Verification items for the finished model (mm, model axes). A direction names the side the tool comes from. Give positions to 0.01 mm unless a question says otherwise; leave off trailing zeros. Loops run counter-clockwise (first coordinate to the right, second up) from the corner with the lowest first, then second, coordinate; pieces in that order, holes last. Notation, with made-up numbers: M 82,-22.5 L 97,-22.5 A36 cw 97,15.5 Z; hole C 1,43.5 d8. An arc over 180 degrees is marked long. Use a Markdown table: item, result.
from build123d import *

# Parameters (mm, degrees)
SKETCH1_R           = 125
BOSS_EXTRUDE1_DEPTH = 6
SKETCH2_R           = 2.5
CUT_EXTRUDE1_DEPTH  = 6
SKETCH3_R           = 12.5
CUT_EXTRUDE2_DEPTH  = 6
SKETCH5_R           = 2.5
CUT_EXTRUDE4_DEPTH  = 10
SKETCH7_R           = 1
CUT_EXTRUDE7_DEPTH  = 10
SKETCH8_R           = 2
CUT_EXTRUDE8_DEPTH  = 10
SKETCH9_R           = 1.25
CUT_EXTRUDE9_DEPTH  = 10
SKETCH10_R          = 8
CUT_EXTRUDE10_DEPTH = 10


with BuildPart() as part:
    # Sketch1 → Boss-Extrude1 (new body)
    with BuildSketch(Plane(origin=(0, 0, 0), x_dir=(1, 0, 0), z_dir=(0, 1, 0))):
        Circle(SKETCH1_R)
    extrude(amount=BOSS_EXTRUDE1_DEPTH)

    # Sketch2 → Cut-Extrude1 (cut)
    with BuildSketch(Plane(origin=(0, 0, 0), x_dir=(1, 0, 0), z_dir=(0, 1, 0))):
        with Locations((0, 110)):
            Circle(SKETCH2_R)
        with Locations((110, 0)):
            Circle(SKETCH2_R)
        with Locations((0, -110)):
            Circle(SKETCH2_R)
        with Locations((-110, 0)):
            Circle(SKETCH2_R)
    extrude(amount=CUT_EXTRUDE1_DEPTH, mode=Mode.SUBTRACT)

    # Sketch3 → Cut-Extrude2 (cut)
    with BuildSketch(Plane(origin=(0, 0, 0), x_dir=(1, 0, 0), z_dir=(0, 1, 0))):
        Circle(SKETCH3_R)
    extrude(amount=CUT_EXTRUDE2_DEPTH, mode=Mode.SUBTRACT)

    # Sketch5 → Cut-Extrude4 (cut)
    with BuildSketch(Plane(origin=(0, 0, 0), x_dir=(1, 0, 0), z_dir=(0, 1, 0))):
        with Locations((17.67766953, 17.67766953)):
            Circle(SKETCH5_R)
        with Locations((-17.67766953, -17.67766953)):
            Circle(SKETCH5_R)
    extrude(amount=CUT_EXTRUDE4_DEPTH, mode=Mode.SUBTRACT)

    # Sketch7 → Cut-Extrude7 (cut)
    with BuildSketch(Plane(origin=(0, 0, 0), x_dir=(1, 0, 0), z_dir=(0, 1, 0))):
        with Locations((33.941125497, -19.091883092)):
            Circle(SKETCH7_R)
        with Locations((19.091883092, -33.941125497)):
            Circle(SKETCH7_R)
        with Locations((25.102290732, -10.253048327)):
            Circle(SKETCH7_R)
        with Locations((10.253048327, -25.102290732)):
            Circle(SKETCH7_R)
        Polygon((33.234018716, -26.870057685), (26.870057685, -33.234018716), (20.506096654, -26.870057685), (26.870057685, -20.506096654), align=None)
    extrude(amount=CUT_EXTRUDE7_DEPTH, mode=Mode.SUBTRACT)

    # Sketch8 → Cut-Extrude8 (cut)
    with BuildSketch(Plane(origin=(0, 0, 0), x_dir=(1, 0, 0), z_dir=(0, 1, 0))):
        with Locations((-11, -110)):
            Circle(SKETCH8_R)
        with Locations((11, -110)):
            Circle(SKETCH8_R)
        with Locations((-110, 11)):
            Circle(SKETCH8_R)
        with Locations((-110, -11)):
            Circle(SKETCH8_R)
        with Locations((11, 110)):
            Circle(SKETCH8_R)
        with Locations((-11, 110)):
            Circle(SKETCH8_R)
        with Locations((110, -11)):
            Circle(SKETCH8_R)
        with Locations((110, 11)):
            Circle(SKETCH8_R)
    extrude(amount=CUT_EXTRUDE8_DEPTH, mode=Mode.SUBTRACT)

    # Sketch9 → Cut-Extrude9 (cut)
    with BuildSketch(Plane(origin=(0, 0, 0), x_dir=(1, 0, 0), z_dir=(0, 1, 0))):
        with Locations((34.825008975, 50.027804771)):
            Circle(SKETCH9_R)
        with Locations((24.218407257, 39.421203053)):
            Circle(SKETCH9_R)
        with Locations((39.421203053, 24.218407258)):
            Circle(SKETCH9_R)
        with Locations((50.027804771, 34.825008975)):
            Circle(SKETCH9_R)
    extrude(amount=CUT_EXTRUDE9_DEPTH, mode=Mode.SUBTRACT)

    # Sketch10 → Cut-Extrude10 (cut)
    with BuildSketch(Plane(origin=(0, 0, 0), x_dir=(1, 0, 0), z_dir=(0, 1, 0))):
        with Locations((-22.627416998, -41.012193309)):
            Circle(SKETCH10_R)
        with Locations((-41.012193309, -22.627416998)):
            Circle(SKETCH10_R)
    extrude(amount=CUT_EXTRUDE10_DEPTH, mode=Mode.SUBTRACT)


solid = part.part
(1) Cross-section at C-C on y = 4. State how many separate pieces and enclosed holes the cut face has, then the cut area to 3 significant figures.
Results below:
| item | result |
|---|---|
| separate pieces | 1 |
| enclosed holes | 26 |
| area | 47,900 mm^2 |
(2) Material ranges on line 1 (X direction, y = 3.5, z = 0); line 2 (X direction, y = 1.3, z = -11); line 3 (Z direction, x = -16.5, y = 0.75), recorded low to high.
Results below:
| item | result |
|---|---|
| line 1 | -125 to -112.5, -107.5 to -12.5, 12.5 to 107.5, 112.5 to 125 |
| line 2 | -124.52 to -112, -108 to -5.94, 5.94 to 108, 112 to 124.52 |
| line 3 | -123.91 to 15.47, 19.88 to 35.87, 46.16 to 123.91 |
(3) Cross-section at B-B on x = -27. Record the cut outline in (y, z).
Results below:
| item | result |
|---|---|
| outline | M 0,-122.05 L 6,-122.05 L 6,34.31 L 0,34.31 Z; M 0,47.71 L 6,47.71 L 6,122.05 L 0,122.05 Z |
(4) Cross-section at D-D on x = 68. Record the cut outline in (y, z), then the cut area to 3 significant figures.
Results below:
| item | result |
|---|---|
| outline | M 0,-104.89 L 6,-104.89 L 6,104.89 L 0,104.89 Z |
| area | 1,260 mm^2 |
(5) Draft check along X on faces 3 (the cylindrical face through (-124.88, 2.96, -5.5)), 4 (the flat face through (-2, 0, 26)), 5 (the flat face through (23.644, 2.958, 23.733)). Enter one of: +X half, -X half, draft (parallel to the pull), parting line (faces both ways), or undercut.
Results below:
| item | result |
|---|---|
| face 3 | parting line |
| face 4 | draft |
| face 5 | undercut |
(6) Gauge pin test, flat ends, axial feed: P1, Ø3, axis at x = -17.5, y = 3.5, coming from the +Z side; P2, Ø3, axis at y = 4, z = 90, coming from the +X side. Record the tip position at first contact, or that the pin passes through.
Results below:
| item | result |
|---|---|
| P1 | z = 123.97 |
| P2 | x = 88.28 |
(7) Set-up check for faces 1 (the flat face through (-2, 6, 26)), 2 (the flat face through (30.007, 2.958, 23.644)): record each of +Z, -Z, +X, -X, +Y, -Y from which the full face is reachable in a straight line by a thin tool's end or side.
Results below:
| item | result |
|---|---|
| face 1 | +Z, -Z, +X, -X, +Y |
| face 2 | +Y, -Y |
(8) Cross-section at A-A on z = -6. Record the cut outline in (x, y).
Results below:
| item | result |
|---|---|
| outline | M -124.86,0 L -10.97,0 L -10.97,6 L -124.86,6 Z; M 10.97,0 L 124.86,0 L 124.86,6 L 10.97,6 Z |
